The model under review builds one solid part; all positions refer to its coordinate system, in mm. A direction names the side the tool comes from. Round coordinates to 2 decimals unless told otherwise and drop trailing zeros. Write each loop counter-clockwise with the first axis right and the second up, starting at its lowest first coordinate (ties: lowest second). Pieces come first, ordered by that corner, then holes. Notation, with made-up numbers: M -36,23.5 L -25,23.5 A13 ccw -25,38.5 Z; hole C -28.5,76.5 d10. An arc over 180 degrees is marked long. Write item = value, one per line. Start each with the question number.
Item 1: Take a section at D-D, the plane y = 7. Give the boundary of the cut face in (x, z).
Item 2: Take a section at A-A, the plane y = 42.5. Give the boundary of the cut face in (x, z).
Item 3: To check wall thickness, follow line 1 along Y through (x, z) = (18, -0.5); line 2 along Y through (x, z) = (-40.5, -3); line 3 along Z through (x, y) = (2.5, 16). State the ranges of each line that lie inside material, in increasing order.
Item 4: The part is to be moulded in two halves that separate along X. For faces 4 (the cylindrical face through (36.75, 1.88, 0.05)), 5 (the flat face through (1, 18, 12)), 6 (the flat face through (31.1, 12, 17)), say which applies: +X half, -X half, draft (parallel to the pull), parting line (faces both ways), or undercut.
Item 5: For pin 1 Ø6 at (x, z) = (-39, 0) entering from +Y; pin 2 Ø7 at (y, z) = (47.5, -4.5) entering from -X; pin 3 Ø1.2 at (x, z) = (29.5, 20) entering from -Y, all flat-tipped, find the tip position at first contact; note any pin that passes through.
Item 6: Take a section at C-C, the plane z = 0. Give the number of separate pieces and of enclosed holes in the cut face, plus the area to 3 significant figures.
Item 7: Tool access review of faces 1 (the flat face through (29, 8.4, 17)), 2 (the flat face through (40, 14, -9)), 3 (the flat face through (-41, 3.7, 2)): name each direction out of +Z, -Z, +X, -X, +Y, -Y from which nothing blocks a thin tool from reaching the whole face with its end or side.
Item 8: Take a section at B-B, the plane x = -39. Give the boundary of the cut face in (y, z).
from build123d import *

# Parameters (mm, degrees)
SKETCH1_W           = 70
SKETCH1_H           = 65
BOSS_EXTRUDE1_DEPTH = 12
BOSS_EXTRUDE2_START = 10
BOSS_EXTRUDE2_DEPTH = 90
BOSS_EXTRUDE3_DEPTH = 3
SKETCH4_W           = 40.5
SKETCH4_H           = 10
BOSS_EXTRUDE4_DEPTH = 13
SKETCH5_W           = 40.5
SKETCH5_H           = 30.5
CUT_EXTRUDE1_DEPTH  = 24
SKETCH6_W           = 4
SKETCH6_H           = 8
BOSS_EXTRUDE5_DEPTH = 11
FILLET1_SIZE        = 3
SKETCH7_R           = 2.25
CUT_EXTRUDE2_DEPTH  = 3.7


with BuildPart() as part:
    # Sketch1 → Boss-Extrude1 (new, symmetric)
    with BuildSketch(Plane.XY):
        with Locations((0, 32.5)):
            Rectangle(SKETCH1_W, SKETCH1_H)
    extrude(amount=BOSS_EXTRUDE1_DEPTH, both=True)

    # Sketch2 → Boss-Extrude2 (add)
    with BuildSketch(Plane(origin=(35, 0, 0), x_dir=(0, 0, -1), z_dir=(1, 0, 0)).offset(BOSS_EXTRUDE2_START)):
        Polygon((12, 20), (12, 0), (-12, 0), (-12, 3.7), (9, 3.7), (9, 20), align=None)
    extrude(amount=-BOSS_EXTRUDE2_DEPTH)

    # Sketch3 → Boss-Extrude3 (add)
    with BuildSketch(Plane(origin=(0, 0, -12), x_dir=(-1, 0, 0), z_dir=(0, 0, -1))):
        Polygon((-45, 20), (-35, 20), (-35, 30), align=None)
        Polygon((35, 30), (45, 20), (35, 20), align=None)
    extrude(amount=-BOSS_EXTRUDE3_DEPTH)

    # Sketch4 → Boss-Extrude4 (add)
    with BuildSketch(Plane.XY.offset(-12)):
        with Locations((0, 55.5)):
            Rectangle(SKETCH4_W, SKETCH4_H)
    extrude(amount=-BOSS_EXTRUDE4_DEPTH)

    # Sketch5 → Cut-Extrude1 (cut)
    with BuildSketch(Plane.XY.offset(12)):
        with Locations((0, 35.25)):
            Rectangle(SKETCH5_W, SKETCH5_H)
    extrude(amount=-CUT_EXTRUDE1_DEPTH, mode=Mode.SUBTRACT)

    # Sketch6 → Boss-Extrude5 (add)
    with BuildSketch(Plane.XY.offset(12)):
        with Locations((29.1, 12.4)):
            Rectangle(SKETCH6_W, SKETCH6_H)
    extrude(amount=BOSS_EXTRUDE5_DEPTH)

    # Fillet1
    # a fillet whose section is not a circle: 3 mm, written as the material it takes off along each edge
    with BuildSketch(Plane(origin=(-35, 65, 19.5), x_dir=(0, -1, 0), z_dir=(0, 0, -1)), Plane(origin=(35, 65, -19.5), x_dir=(0, -1, 0), z_dir=(0, 0, 1))) as fillet1_piece_1:
        with BuildLine():
            Bezier((FILLET1_SIZE, 0), (0, 0), (0, -FILLET1_SIZE), weights=[1, 0.428571429, 1])
            Line((0, -FILLET1_SIZE), (0, 0))
            Line((0, 0), (FILLET1_SIZE, 0))
        make_face()
    extrude(amount=39, mode=Mode.SUBTRACT)
    with BuildSketch(Plane(origin=(-20.25, 43, -25), x_dir=(0, 0, 1), z_dir=(0, 1, 0)), Plane(origin=(20.25, 68, -25), x_dir=(0, 0, 1), z_dir=(0, -1, 0))) as fillet1_piece_2:
        with BuildLine():
            Bezier((FILLET1_SIZE, 0), (0, 0), (0, FILLET1_SIZE), weights=[1, 0.428571429, 1])
            Line((0, FILLET1_SIZE), (0, 0))
            Line((0, 0), (FILLET1_SIZE, 0))
        make_face()
    extrude(amount=25, mode=Mode.SUBTRACT)

    # Sketch7 → Cut-Extrude2 (cut)
    with BuildSketch(Plane(origin=(0, 3.7, 0), x_dir=(1, 0, 0), z_dir=(0, 1, 0))):
        with Locations(Location((-39, 0, 0), (0, 0, 270))):
            Circle(SKETCH7_R)
        with BuildLine():
            Line((39, 2.25), (40, 2.25))
            ThreePointArc((40, 2.25), (42.25, 0), (40, -2.25))
            Line((40, -2.25), (39, -2.25))
            ThreePointArc((39, -2.25), (36.75, 0), (39, 2.25))
        make_face()
    extrude(amount=-CUT_EXTRUDE2_DEPTH, mode=Mode.SUBTRACT)


solid = part.part
Response values:
q1.outline = M -45,-12 L 45,-12 L 45,-9 L 35,-9 L 35,12 L -35,12 L -35,-9 L -45,-9 Z
q2.outline = M -35,-12 L -20.25,-12 L -20.25,12 L -35,12 Z; M 20.25,-12 L 35,-12 L 35,12 L 20.25,12 Z
q3.line_1 = 0 to 20, 50.5 to 65
q3.line_2 = 0 to 3.7
q3.line_3 = -12 to 12
q4.face_4 = undercut
q4.face_5 = draft
q4.face_6 = +X half
q5.pin_1 = 3.7
q5.pin_2 = -35
q5.pin_3 = 8.4
q6.separate_pieces = 3
q6.enclosed_holes = 1
q6.area = 3,350 mm2
q7.face_1 = +Z, +X, -X, -Y
q7.face_2 = +Z, +X, +Y
q7.face_3 = +Z, -X, +Y
q8.outline = M 0,-12 L 26,-12 L 26,-9 L 3.7,-9 L 3.7,-2.25 L 0,-2.25 Z; M 0,2.25 L 3.7,2.25 L 3.7,12 L 0,12 Z
